The model under review builds one solid part; all positions refer to its coordinate system, in mm. A direction names the side the tool comes from. Coordinates: 2 decimals unless noted, no trailing zeros. Loops run counter-clockwise (first coordinate to the right, second up) from the corner with the lowest first, then second, coordinate; pieces in that order, holes last. Notation, with made-up numbers: (32, 38.25) - (68, 38.25) arc R23 cw to (68, 73.25) - close; hole circle Ø3 at (0.25, -39.75). An arc over 180 degrees is marked (long way). One line per item, written item: value. Start each with the question number.
1. Insertion check: P1, Ø2.5, axis at y = -2, z = -19, coming from the +X side; P2, Ø1.5, axis at x = 33.5, y = -3.5, coming from the +Z side; P3, Ø2, axis at x = 0, z = 0, coming from the +Y side; P4, Ø1.5, axis at x = 39, y = -3.5, coming from the -Z side. Each pin has a flat end and moves straight along its axis. Give the tip position at first contact, or say it passes through.
2. For faces 1 (the face through (-5, -2, 16)), 2 (the face through (-5, -2, -17)), 3 (the face through (109.6, -2.46, 0.06)), 4 (the face through (-15, -2, 0)), list the 3-axis set-ups (+Z, -Z, +X, -X, +Y, -Y) from which the entire face can be reached by the end or side of a thin tool; tool diameter is ignored.
3. We need section C-C, the plane x = 111. Give the boundary of the cut face in (y, z), then the cut area to 3 significant figures.
4. Mouldability with a two-part tool opening along Z and no side actions: class faces 5 (the face through (-1.4, -2.46, 0.06)), 6 (the face through (58, -2, 5)), 7 (the face through (-14, -2, -25)), 8 (the face through (33, -5, 0)) as +Z half, -Z half, draft (parallel to the pull), parting line (faces both ways), or undercut.
5. We need section D-D, the plane x = 15.5. Give the boundary of the cut face in (y, z).
6. To check wall thickness, follow line 1 (Z direction, x = 111, y = -1.8); line 2 (Z direction, x = 49, y = -4.65); line 3 (X direction, y = -0.9, z = 11). State the ranges of each line that lie inside material, in increasing order.
7. We need section B-B, the plane z = 0. Give the boundary of the cut face in (x, y).
8. We need section A-A, the plane y = -3.45. Give the boundary of the cut face in (x, z).
from build123d import *

# Parameters (mm, degrees)
F0_R     = 1.4
F1_DEPTH = 5


with BuildPart() as f1:
    # F0 (on Front) → F1 (new body)
    with BuildSketch(Plane.XZ):
        with BuildLine():
            ThreePointArc((-5, -10), (-3.535534, -6.464466), (0, -5))
            Line((0, -5), (114, -5))
            ThreePointArc((114, -5), (115.414214, -4.414214), (116, -3))
            Line((116, -3), (116, 3))
            ThreePointArc((116, 3), (115.414214, 4.414214), (114, 5))
            Line((114, 5), (0, 5))
            ThreePointArc((0, 5), (-3.535534, 6.464466), (-5, 10))
            Line((-5, 10), (-5, 23))
            ThreePointArc((-5, 23), (-5.585786, 24.414214), (-7, 25))
            Line((-7, 25), (-15, 25))
            Line((-15, 25), (-20, 25))
            Line((-20, 25), (-20, 15))
            Line((-20, 15), (-15, 15))
            Line((-15, 15), (-15, -15))
            Line((-15, -15), (-20, -15))
            Line((-20, -15), (-20, -25))
            Line((-20, -25), (-15, -25))
            Line((-15, -25), (-7, -25))
            ThreePointArc((-7, -25), (-5.585786, -24.414214), (-5, -23))
            Line((-5, -23), (-5, -10))
        make_face()
        Circle(F0_R, mode=Mode.SUBTRACT)
        with Locations((111, 0)):
            Circle(F0_R, mode=Mode.SUBTRACT)
    extrude(amount=F1_DEPTH)


solid = f1.part
Findings below:
1. P1: x = -5
1. P2: z = 5
1. P3: through
1. P4: z = -5
2. face 1: +Z, +X, +Y, -Y
2. face 2: -Z, +X, +Y, -Y
2. face 3: +Y, -Y
2. face 4: -X, +Y, -Y
3. outline: (-5, -5) - (0, -5) - (0, -1.4) - (-5, -1.4) - close; (-5, 1.4) - (0, 1.4) - (0, 5) - (-5, 5) - close
3. area: 36.0 mm2
4. face 5: undercut
4. face 6: +Z half
4. face 7: -Z half
4. face 8: draft
5. outline: (-5, -5) - (0, -5) - (0, 5) - (-5, 5) - close
6. line 1: -5 to -1.4, 1.4 to 5
6. line 2: -5 to 5
6. line 3: -15 to -5
7. outline: (-15, -5) - (-1.4, -5) - (-1.4, 0) - (-15, 0) - close; (1.4, -5) - (109.6, -5) - (109.6, 0) - (1.4, 0) - close; (112.4, -5) - (116, -5) - (116, 0) - (112.4, 0) - close
8. outline: (-20, -25) - (-7, -25) arc R2 ccw to (-5, -23) - (-5, -10) arc R5 cw to (0, -5) - (114, -5) arc R2 ccw to (116, -3) - (116, 3) arc R2 ccw to (114, 5) - (0, 5) arc R5 cw to (-5, 10) - (-5, 23) arc R2 ccw to (-7, 25) - (-20, 25) - (-20, 15) - (-15, 15) - (-15, -15) - (-20, -15) - close; hole circle Ø2.8 at (0, 0); hole circle Ø2.8 at (111, 0)
